Here's how the part is built. I have some questions about the finished solid (model axes, mm). Give positions to 0.01 mm unless a question says otherwise; leave off trailing zeros. Write each loop counter-clockwise with the first axis right and the second up, starting at its lowest first coordinate (ties: lowest second). Pieces come first, ordered by that corner, then holes. Notation, with made-up numbers: (71.25, -27) -> (113.25, -27) arc R20 ccw to (113.25, 4) -> close; hole circle Ø7 at (21, 67.25). An arc over 180 degrees is marked (long way). Return JSON: item names as keys, results as strings.
from build123d import *

# Parameters (mm, degrees)
F0_W     = 38.1
F0_H     = 38.1
F1_DEPTH = 2.54
F2_R     = 5.715
F3_DEPTH = 25.4
F4_R     = 1.5875
F5_DEPTH = 25.4


with BuildPart() as f1:
    # F0 (on Top) → F1 (new body)
    with BuildSketch(Plane.XY):
        Rectangle(F0_W, F0_H)
    extrude(amount=F1_DEPTH)

    # F2 (on Top) → F3 (cut)
    with BuildSketch(Plane.XY):
        Circle(F2_R)
    extrude(amount=F3_DEPTH, mode=Mode.SUBTRACT)

    # F4 (on Top) → F5 (cut)
    with BuildSketch(Plane.XY):
        with Locations((13.97, 13.97)):
            Circle(F4_R)
    extrude(amount=F5_DEPTH, mode=Mode.SUBTRACT)

    # F6: F1 across plane


with BuildPart() as f1_1:
    add(f1.part)
    add(f1.part.mirror(Plane.YZ), mode=Mode.INTERSECT)

    # F7: F1 across plane


with BuildPart() as f1_2:
    add(f1_1.part)
    add(f1_1.part.mirror(Plane.XZ), mode=Mode.INTERSECT)


solid = f1_2.part
1. Suppose I cut it at A-A, the plane x = 0. List the corners of the cut face in (y, z) for me (3 decimals), and give its area (3 significant figures).
Taken from the geometry:
{"outline": "(-19.05, 0) -> (-5.715, 0) -> (-5.715, 2.54) -> (-19.05, 2.54) -> close; (5.715, 0) -> (19.05, 0) -> (19.05, 2.54) -> (5.715, 2.54) -> close", "area": "67.7 mm²"}
2. If I drill on line 1 (X direction, y = -13.97, z = 1.7); line 2 (Y direction, x = -15, z = 1.9), over which ranges is the centre line in solid material (lowest first)? Write a range as [from, to].
Taken from the geometry:
{"line 1": "x = [-19.05, -15.56], [-12.38, 12.38], [15.56, 19.05]", "line 2": "y = [-19.05, -15.18], [-12.76, 12.76], [15.18, 19.05]"}
3. Suppose I cut it at D-D, the plane z = 1.25. Count the separate pieces of the cut face and the enclosed holes in it, and give its area (3 significant figures).
Taken from the geometry:
{"separate pieces": "1", "enclosed holes": "5", "area": "1,320 mm²"}
4. Suppose I cut it at B-B, the plane y = 13.97. List the corners of the cut face in (x, z) for me, and give its area (3 significant figures).
Taken from the geometry:
{"outline": "(-19.05, 0) -> (-15.56, 0) -> (-15.56, 2.54) -> (-19.05, 2.54) -> close; (-12.38, 0) -> (12.38, 0) -> (12.38, 2.54) -> (-12.38, 2.54) -> close; (15.56, 0) -> (19.05, 0) -> (19.05, 2.54) -> (15.56, 2.54) -> close", "area": "80.6 mm²"}
5. If we mould it in two halves opening along X, with no side actions, what happens to faces 1 (the face through (15.436, 13.362, 1.252)), 2 (the face through (19.05, 0, 1)), 3 (the face through (4, 5, 2.54))? For each: released by +X, released by -X, zero draft, split by the parting line, or undercut.
Taken from the geometry:
{"face 1": "undercut", "face 2": "released by +X", "face 3": "zero draft"}
6. For pin 1 Ø18.5 at (x, y) = (0, 0) entering from +Z, with a flat end and sliding along its axis, tell me the tip position at first contact or that it passes through.
Taken from the geometry:
{"pin 1": "stops at z = 2.54"}
